For this review, use the dimensioned drawing (mm, ordinates from the lowest corner) and the shaded views. A direction names the side the tool comes from. Coordinates: 2 decimals unless noted, no trailing zeros. Loops run counter-clockwise (first coordinate to the right, second up) from the corner with the lowest first, then second, coordinate; pieces in that order, holes last. Notation, with made-up numbers: M 71.25,49.25 L 99.25,49.25 A14 ccw 99.25,72.25 Z; hole C 53,89.5 d6. An arc over 180 degrees is marked long. Write item = value, one per line. Start each with the question number.
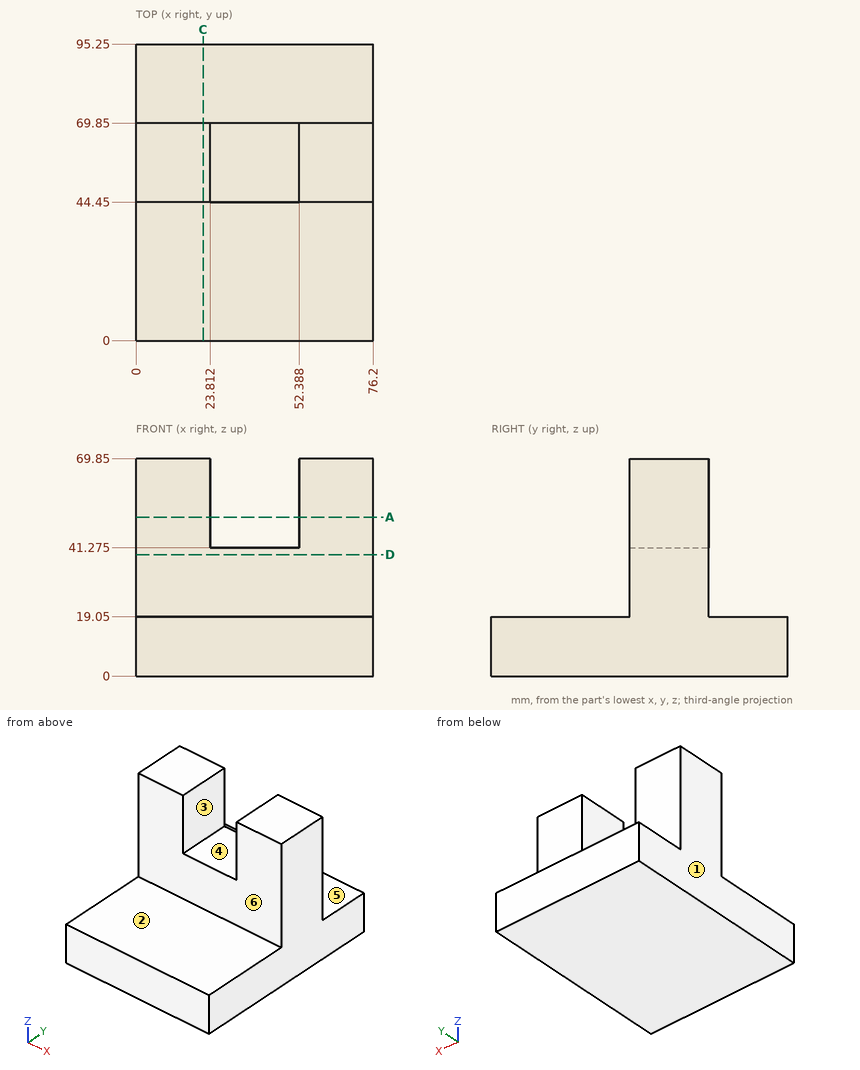
Q1. Add section A-A on z = 51. State the section outline as (x, y) points.
Q2. Mouldability with a two-part tool opening along X and no side actions: class the marked faces 1, 2 and 3 as released by +X, released by -X, zero draft, split by the parting line, or undercut.
Q3. To check wall thickness, follow line 1 (X direction, y = 64.5, z = 46); line 2 (Z direction, x = 62.5, y = 14.5); line 3 (Z direction, x = 36.5, y = 64.5) (1 decimal). State the ranges of each line that lie inside material, in increasing order. Write a range as from..to.
Q4. For the marked faces 4, 5 and 6, list the 3-axis set-ups (+Z, -Z, +X, -X, +Y, -Y) from which the entire face can be reached by the end or side of a thin tool; tool diameter is ignored.
Q5. Add section D-D on z = 39. State the section outline as (x, y) points, plus the area to 3 significant figures.
Q6. Add section C-C on x = 21.5. State the section outline as (y, z) points.
Q7. Clearance check with flat-ended pins moving along their axes: P1, Ø20.5, axis at x = 42.5, y = 87, coming from the +Z side; P2, Ø12, axis at x = 62.5, z = 27, coming from the -Y side; P3, Ø7.5, axis at x = 37.5, y = 57.5, coming from the +Z side (1 decimal). State where each tip first meets the part, or that it passes through.
Values follow:
q1.outline = M 0,44.45 L 23.81,44.45 L 23.81,69.85 L 0,69.85 Z; M 52.39,44.45 L 76.2,44.45 L 76.2,69.85 L 52.39,69.85 Z
q2.face_1 = released by -X
q2.face_2 = zero draft
q2.face_3 = undercut
q3.line_1 = 0..23.81, 52.39..76.2
q3.line_2 = 0..19.05
q3.line_3 = 0..41.3
q4.face_4 = +Z, +Y, -Y
q4.face_5 = +Z, +X, -X, +Y
q4.face_6 = +Z, +X, -X, -Y
q5.outline = M 0,44.45 L 76.2,44.45 L 76.2,69.85 L 0,69.85 Z
q5.area = 1,940 mm2
q6.outline = M 0,0 L 95.25,0 L 95.25,19.05 L 69.85,19.05 L 69.85,69.85 L 44.45,69.85 L 44.45,19.05 L 0,19.05 Z
q7.P1 = 19.05
q7.P2 = 44.45
q7.P3 = 41.3
